from build123d import *

# Parameters (mm, degrees)
BOSS_EXTRUDE2_DEPTH = 10


with BuildPart() as part:
    # Sketch1 → Boss-Extrude2 (new, symmetric)
    with BuildSketch(Plane.XY):
        with BuildLine():
            Line((-28.85, 13.3), (20.15, 13.3))
            Line((20.15, 13.3), (20.15, 12.1))
            Line((20.15, 12.1), (-28.85, 12.1))
            ThreePointArc((-28.85, 12.1), (-29.132842712, 11.982842712), (-29.25, 11.7))
            Line((-29.25, 11.7), (-29.25, 1))
            ThreePointArc((-29.25, 1), (-29.132842712, 0.717157288), (-28.85, 0.6))
            Line((-28.85, 0.6), (28.85, 0.6))
            ThreePointArc((28.85, 0.6), (29.132842712, 0.717157288), (29.25, 1))
            Line((29.25, 1), (29.25, 13))
            ThreePointArc((29.25, 13), (29.132842712, 13.282842712), (28.85, 13.4))
            Line((28.85, 13.4), (-30.15, 13.4))
            ThreePointArc((-30.15, 13.4), (-30.432842712, 13.282842712), (-30.55, 13))
            Line((-30.55, 13), (-30.55, -0.3))
            ThreePointArc((-30.55, -0.3), (-30.432842712, -0.582842712), (-30.15, -0.7))
            Line((-30.15, -0.7), (30.15, -0.7))
            ThreePointArc((30.15, -0.7), (30.432842712, -0.582842712), (30.55, -0.3))
            Line((30.55, -0.3), (30.55, 8.7))
            Line((30.55, 8.7), (31.75, 8.7))
            Line((31.75, 8.7), (31.75, -0.3))
            ThreePointArc((31.75, -0.3), (31.28137085, -1.43137085), (30.15, -1.9))
            Line((30.15, -1.9), (-30.15, -1.9))
            ThreePointArc((-30.15, -1.9), (-31.28137085, -1.43137085), (-31.75, -0.3))
            Line((-31.75, -0.3), (-31.75, 13))
            ThreePointArc((-31.75, 13), (-31.28137085, 14.13137085), (-30.15, 14.6))
            Line((-30.15, 14.6), (28.85, 14.6))
            ThreePointArc((28.85, 14.6), (29.98137085, 14.13137085), (30.45, 13))
            Line((30.45, 13), (30.45, 1))
            ThreePointArc((30.45, 1), (29.98137085, -0.13137085), (28.85, -0.6))
            Line((28.85, -0.6), (-28.85, -0.6))
            ThreePointArc((-28.85, -0.6), (-29.98137085, -0.13137085), (-30.45, 1))
            Line((-30.45, 1), (-30.45, 11.7))
            ThreePointArc((-30.45, 11.7), (-29.98137085, 12.83137085), (-28.85, 13.3))
        make_face()
    extrude(amount=BOSS_EXTRUDE2_DEPTH, both=True)


solid = part.part
Here's how the part is built. I have some questions about the finished solid (model axes, mm). A direction names the side the tool comes from. Round coordinates to 2 decimals unless told otherwise and drop trailing zeros. Write each loop counter-clockwise with the first axis right and the second up, starting at its lowest first coordinate (ties: lowest second). Pieces come first, ordered by that corner, then holes. Notation, with made-up numbers: (59, 64.5) -> (64, 64.5) arc R34 cw to (64, 95.5) -> close; hole circle Ø4 at (40, -22.75). An arc over 180 degrees is marked (long way). One line per item, written item: value.
1) We'd pull the mould along Y, two halves only. Please class faces 1 (the face through (31, 8.7, 0)), 2 (the face through (29.25, 7, 0)), 3 (the face through (-2, 0, -10)): released by +Y, released by -Y, zero draft, split by the parting line, or undercut.
Filled sheet:
face 1: released by +Y
face 2: undercut
face 3: zero draft
2) Suppose I cut it at A-A on y = 2.75. List the corners of the cut face in (x, z) for me, plus the area to 3 significant figures.
Filled sheet:
outline: (-31.75, -10) -> (-30.55, -10) -> (-30.55, 10) -> (-31.75, 10) -> close; (-30.45, -10) -> (-29.25, -10) -> (-29.25, 10) -> (-30.45, 10) -> close; (29.25, -10) -> (30.45, -10) -> (30.45, 10) -> (29.25, 10) -> close; (30.55, -10) -> (31.75, -10) -> (31.75, 10) -> (30.55, 10) -> close
area: 96.0 mm2
3) Suppose I cut it at B-B on x = 18.5. List the corners of the cut face in (y, z) for me.
Filled sheet:
outline: (-1.9, -10) -> (-0.7, -10) -> (-0.7, 10) -> (-1.9, 10) -> close; (-0.6, -10) -> (0.6, -10) -> (0.6, 10) -> (-0.6, 10) -> close; (12.1, -10) -> (13.3, -10) -> (13.3, 10) -> (12.1, 10) -> close; (13.4, -10) -> (14.6, -10) -> (14.6, 10) -> (13.4, 10) -> close
4) If I drill on line 1 (X direction, y = 12.75, z = 3.25); line 2 (X direction, y = -1, z = -2.5); line 3 (X direction, y = -0.75, z = 5.5), over which ranges is the centre line in solid material (lowest first)? Write a range as [from, to].
Filled sheet:
line 1: x = [-31.75, -30.55], [-30.06, 20.15], [29.25, 30.45]
line 2: x = [-31.59, 31.59]
line 3: x = [-31.69, 31.69]
5) For faces 4 (the face through (31.75, 4, 0)), 5 (the face through (-29.99, 12.82, 0.14)), which set-ups out of +Z, -Z, +X, -X, +Y, -Y let a thin tool reach every point of the face, with its end or its side?
Filled sheet:
face 4: +Z, -Z, +X, +Y, -Y
face 5: +Z, -Z
6) I'm going to push flat-ended pins straight in: pin 1 Ø1.3 at (y, z) = (12.5, 4.5) entering from +X; pin 2 Ø3 at (x, y) = (1, 10) entering from +Z. Where does each tip first touch, or does it pass through?
Filled sheet:
pin 1: stops at x = 30.45
pin 2: passes through
